Autodesk Inventor part; units mm, degrees
ref_plane "Work Plane1" through (-108.1719, 0, -146.2869) normal (0, 1, 0) x (0.6910823, 0, -0.7227761)
ref_plane "Work Plane2" through (-186.5657, -6, -277.4707) normal (0.6910823, 0, -0.7227761) x (0, 1, 0)
ref_plane "Work Plane3" through (-14.1966, -8.9, -56.4323) normal (-0.6910823, 0, 0.7227761) x (0.7227761, 0, 0.6910823)
sketch "Sketch1" plane through (0, 0, 0) normal (0, 1, 0) x (-1, 0, 0)
  line L0 (0, 0) -> (100, 0)
  line L1 (100, 0) -> (100, -50)
  line L2 (100, -50) -> (0, -50)
  line L3 (0, -50) -> (0, 0)
  dimension "d0" = 100
  dimension "d1" = 50
extrude "Extrusion1" add sketch "Sketch1" along normal blind 3
sketch "Sketch2" plane through (0, 3, 0) normal (0, 1, 0) x (1, 0, 0)
  circle A0 centre (-85, 25) radius 7
  circle A1 centre (-30, 25) radius 7
  line L0 (-100, 50) -> (-100, 0)
  line L1 (0, 0) -> (0, 50)
  line L2 (0, 50) -> (-100, 50)
  dimension "d4" = 14
  dimension "d5" = 14
  dimension "d6" = 15
  dimension "d7" = 30
  dimension "d8" = 25
  dimension "d9" = 25
extrude "Extrusion2" add sketch "Sketch2" along normal blind 18
sketch "Sketch3" plane through (-85, 21, -25) normal (0, 1, 0) x (1, 0, 0)
  circle A0 centre (0, 0) radius 7
  circle A1 centre (55, 0) radius 7
  circle A2 centre (0, 0) radius 2.875
  circle A3 centre (55, 0) radius 2.45
  point P0 (85, -25)
  dimension "d12" = 5.75
  dimension "d13" = 4.9
extrude "Extrusion3" add sketch "Sketch3" along normal blind 3 contours A2 | A3
sketch "Sketch5" plane through (-30, 24, -25) normal (0, 1, 0) x (1, 0, 0)
  circle A0 centre (0, 0) radius 1.925
  point P0 (30, -25)
  dimension "d20" = 3.85
extrude "Extrusion5" cut sketch "Sketch5" against normal up to surface (24 mm away)
sketch "Sketch7" plane through (0, 0, 0) normal (0, -1, 0) x (1, 0, 0)
  line L0 (2.4404, 5.5552) -> (-105.2601, 5.5552)
  line L1 (-105.2601, 5.5552) -> (-105.2601, -59.9514)
  line L2 (-105.2601, -59.9514) -> (2.4404, -59.9514)
  line L3 (2.4404, -59.9514) -> (2.4404, 5.5552)
  circle A0 centre (-30, -25) radius 2.45
  circle A1 centre (-30, -25) radius 7
  point P0 (0, 0)
extrude "Extrusion6" cut sketch "Sketch7" against normal blind 50 contours L3 L2 L1 L0
ref_plane "Work Plane1" through (-108.1719, 0, -146.2869) normal (0, 1, 0) x (0.6910823, 0, -0.7227761)
sketch "Sketch8" plane through (-108.1719, 0, -146.2869) normal (0, 1, 0) x (0.6910823, 0, -0.7227761)
  line L0 (-40.64, -147.32) -> (40.64, -147.32)
  line L1 (-40.64, 147.32) -> (-40.64, -147.32)
  line L2 (-43.34, -130.02) -> (-40.84, -130.02)
  line L3 (-40.84, -130.02) -> (-40.84, -150.02)
  line L4 (-40.84, -150.02) -> (-43.34, -150.02)
  line L5 (-43.34, -150.02) -> (-43.34, -130.02)
  line L6 (-23.34, -147.52) -> (-40.84, -147.52)
  line L7 (-40.84, -147.52) -> (-40.84, -150.02)
  line L8 (-23.34, -147.52) -> (-23.34, -150.02)
  line L9 (-23.34, -150.02) -> (-40.84, -150.02)
  line L10 (-40.84, -130.02) -> (-23.34, -130.02)
  line L11 (-23.34, -130.02) -> (-23.34, -147.52)
  arc A0 (-33.6873, -142.3194) -> (-35.0746, -141.7135) centre (-33.64, -140.32) ccw
  circle A1 centre (-33.64, -140.32) radius 3.8
  circle A2 centre (-33.64, -140.32) radius 7
  point P0 (-30.9769, -179.2803)
  point P1 (-40.84, -150.02)
  dimension "d26" = 0.2
  dimension "d27" = 0.2
  dimension "d29" = 20
  dimension "d30" = 2.5
  dimension "d31" = 2.5
  dimension "d32" = 20
extrude "Extrusion7" add sketch "Sketch8" along normal blind 2.5 contours L1 A2 L0 | L0 L11 L6 L3 L10 L1 | A2 L1 L10 L11 L0 | L8 L9 L3 L6 | L3 L4 L5 L2
sketch "Sketch9" plane through (0, 0, 0) normal (0, -1, 0) x (1, 0, 0)
  line L0 (-29.6926, -11.2856) -> (-15.8709, -25.7411)
  line L1 (-15.8709, -25.7411) -> (-17.6779, -27.4688)
  line L2 (-15.8709, -25.7411) -> (-30.3264, -39.5627)
  line L3 (-17.6779, -27.4688) -> (-31.4995, -13.0133)
  line L4 (-30.3264, -39.5627) -> (-44.1481, -25.1072)
  line L5 (-44.1481, -25.1072) -> (-42.4204, -26.9142)
  line L6 (-42.4204, -26.9142) -> (-29.7718, -14.8202)
  line L7 (-30.3264, -39.5627) -> (-44.1481, -25.1072)
  line L8 (-15.8709, -25.7411) -> (-30.3264, -39.5627)
  line L9 (-29.6926, -11.2856) -> (-15.8709, -25.7411)
  line L10 (-44.1481, -25.1072) -> (-29.6926, -11.2856)
  circle A0 centre (-30, -25) radius 1.925
  point P0 (0, 0)
  dimension "d35" = 2.5
  dimension "d36" = 0
  dimension "d37" = 2.5
extrude "Extrusion8" add sketch "Sketch9" along normal blind 6.4 contours L0 L1 L3 L10 | L3 L6 L4 L10
sketch "Sketch10" plane through (0, -6.4, 0) normal (0, -1, 0) x (1, 0, 0)
  line L0 (-30.3264, -39.5627) -> (-44.1481, -25.1072)
  line L1 (-44.1481, -25.1072) -> (-29.6926, -11.2856)
  line L2 (-29.6926, -11.2856) -> (-15.8709, -25.7411)
  line L3 (-15.8709, -25.7411) -> (-30.3264, -39.5627)
  circle A0 centre (-30, -25) radius 7
  circle A1 centre (-30, -25) radius 1.925
  point P0 (0, 0)
extrude "Extrusion9" add sketch "Sketch10" along normal blind 2.5 contours L0 L1 L2 L3 | A0
fillet "Fillet1" radius 2.5 1 edges at (-29.6926, -3.2, -11.2856)
fillet "Fillet2" radius 2.5 1 edges at (-37, 2.5, -25)
sketch "Sketch11" plane through (0, -8.9, 0) normal (0, -1, 0) x (1, 0, 0)
  circle A0 centre (-30, -25) radius 1.925
  arc A1 (-27.9649, -13.0925) -> (-31.4995, -13.0133) centre (-29.7718, -14.8202) ccw
  line L0 (-31.4995, -13.0133) -> (-44.1481, -25.1072)
  line L1 (-44.1481, -25.1072) -> (-30.3264, -39.5627)
  line L2 (-30.3264, -39.5627) -> (-15.8709, -25.7411)
  line L3 (-15.8709, -25.7411) -> (-27.9649, -13.0925)
  circle A2 centre (-30, -25) radius 2.45
  line L4 (-31.3275, -29.5443) -> (-34.5993, -26.1225)
  line L5 (-34.5993, -26.1225) -> (-33.2718, -21.5782)
  line L6 (-33.2718, -21.5782) -> (-28.6725, -20.4557)
  line L7 (-28.6725, -20.4557) -> (-25.4007, -23.8775)
  line L8 (-25.4007, -23.8775) -> (-26.7282, -28.4218)
  line L9 (-26.7282, -28.4218) -> (-31.3275, -29.5443)
  line L10 (-15.8709, -25.7411) -> (-27.9649, -13.0925)
  point P0 (0, 0)
  dimension "d44" = 8.2
extrude "Extrusion10" cut sketch "Sketch11" against normal blind 1.5 contours L4 L5 L6 L7 L8 L9
sketch "Sketch12" plane through (-30.3264, 0, -39.5627) normal (0.6910823, 0, -0.7227761) x (-0.7227761, 0, -0.6910823)
  line L0 (-17.5, 0) -> (0, 0)
  line L1 (0, 0) -> (0, 2.5)
  line L2 (-20, 2.5) -> (0, 2.5)
  line L3 (-20, -8.9) -> (-20, 2.5)
  line L4 (0, -8.9) -> (-20, -8.9)
  line L5 (0, -6.4) -> (0, -8.9)
  line L6 (0, -6.4) -> (-17.5, -6.4)
  line L7 (-17.5, 0) -> (-17.5, -6.4)
  point P0 (-49.2603, 0)
ref_plane "Work Plane2" through (-186.5657, -6, -277.4707) normal (0.6910823, 0, -0.7227761) x (0, 1, 0)
extrude "Extrusion11" add sketch "Sketch12" along normal blind 64.18
sketch "Sketch13" plane through (14.0272, 0, -85.9505) normal (0.6910823, 0, -0.7227761) x (-0.7227761, 0, -0.6910823)
  line L0 (0, 2.5) -> (-17.5, 2.5)
  line L1 (-17.5, -8.9) -> (0, -8.9)
  line L2 (0, -8.9) -> (0, 2.5)
  line L3 (-20, -8.9) -> (-20, 2.5)
  line L4 (-17.5, -6.4) -> (-17.5, 0)
  line L5 (-17.5, 0) -> (0, 0)
  line L6 (0, 0) -> (0, 2.5)
  line L7 (0, 2.5) -> (-20, 2.5)
  line L8 (-20, 2.5) -> (-20, -8.9)
  line L9 (-20, -8.9) -> (0, -8.9)
  line L10 (0, -8.9) -> (0, -6.4)
  line L11 (0, -6.4) -> (-17.5, -6.4)
  point P0 (-49.2603, 0)
  point P1 (-20, 2.5)
extrude "Extrusion12" add sketch "Sketch13" along normal blind 2.5
fillet "Fillet3" radius 2.5 1 edges at (30.2104, -3.2, -73.9358)
ref_plane "Work Plane3" through (-14.1966, -8.9, -56.4323) normal (-0.6910823, 0, 0.7227761) x (0.7227761, 0, 0.6910823)
mirror "Mirror1" about plane through (-14.1966, -8.9, -56.4323) normal (-0.6910823, 0, 0.7227761)
sketch "Sketch14" plane through (16.496, 24, -73.6284) normal (0, 1, 0) x (1, 0, 0)
  circle A0 centre (0, 0) radius 1.925
  circle A1 centre (0, 0) radius 1.925
  circle A2 centre (0, 0) radius 2.45
  point P0 (-16.496, -73.6284)
ref_plane "Work Plane4" through (-246.9785, 21, -281.7123) normal (0, -1, 0) x (0.7227761, 0, 0.6910823)
extrude "Extrusion13" cut sketch "Sketch14" against normal up to surface (3 mm away)
sketch "Sketch15" plane through (16.496, 21, -73.6284) normal (0, 1, 0) x (1, 0, 0)
  circle A0 centre (0, 0) radius 7
  point P0 (-16.496, -73.6284)
ref_plane "Work Plane5" through (-242.7369, 0, -277.4707) normal (0, 1, 0) x (-0.6910823, 0, 0.7227761)
extrude "Extrusion14" add sketch "Sketch15" against normal up to surface (21 mm away)
extrude "Extrusion15" cut sketch "Sketch11" against normal blind 1.5 contours A0 | A2 | L4 L5 L6 L7 L8 L9
extrude "Extrusion16" cut sketch "Sketch5" against normal up to surface (32.9 mm away)
properties part number "Base"
Build history of the part. All positions in model axes, mm. A direction names the side the tool comes from. Give positions to 0.01 mm unless a question says otherwise; leave off trailing zeros. Loops run counter-clockwise (first coordinate to the right, second up) from the corner with the lowest first, then second, coordinate; pieces in that order, holes last. Notation, with made-up numbers: (34, 5) -> (91, 5) arc R25 cw to (91, 28) -> close; hole circle Ø6 at (34, -25.75). An arc over 180 degrees is marked (long way). One line per question, with ' | ' between items. Start each with the question number.
1) Cut at A-A (x = -14.5). Give the cut face in (y, z).
2) Probe L1, parallel to Z at x = -30, y = 17.5 (3 decimals); L2, parallel to X at y = 15, z = -25 (3 decimals); L3, parallel to Y at x = -10.5, z = -46.5. List the from-to ranges inside material, lowest first.
3) Two-plate mould, pull along Y, no slides. Class faces 4 (the flat face through (-8, -6.4, -50)), 5 (the cylindrical face through (-27.663, 22.479, -24.264)), 6 (the flat face through (-7, -8.9, -49)): released by +Y, released by -Y, zero draft, split by the parting line, or undercut.
4) Cut at C-C (z = -36). Give the cut face in (x, y).
5) 3-axis set-ups, long thin cutter, end or side, ignore diameter. For faces 1 (the cylindrical face through (-26.77, 12.89, -31.21)), 2 (the flat face through (20.44, -3.16, -79.82)), 3 (the flat face through (-32.1, -7.4, -24.9)): which of +Z, -Z, +X, -X, +Y, -Y reach the whole face in a straight line?
6) Cut at B-B (y = 11.5). Give the cut face in (x, z) (3 decimals).
7) Pin check, flat tips, straight feed: pin 1 (8 mm diameter, centred on y = 8.5, z = -22, fed in from +X); pin 2 (4 mm diameter, centred on y = 9, z = -74.5, fed in from +X); pin 3 (1 mm diameter, centred on y = -4, z = -58.5, fed in from -X). Stop position of each tip, or through.
Return value:
1) outline: (-8.9, -56.11) -> (-6.4, -56.11) -> (-6.4, -30.79) -> (0, -30.79) -> (0, -56.12) -> (2.5, -56.11) -> (2.5, -27.17) -> (-8.9, -27.17) -> close
2) L1: -32 to -26.925, -23.075 to -18 | L2: -37 to -31.925, -28.075 to -23 | L3: -8.9 to -6.4, 0 to 2.5
3) face 4: undercut | face 5: zero draft | face 6: released by -Y
4) outline: (-33.73, -8.9) -> (-6.06, -8.9) -> (-6.06, 2.5) -> (-33.73, 2.5) -> (-33.73, 0) -> (-9.52, 0) -> (-9.52, -6.4) -> (-33.73, -6.4) -> close
5) face 1: +Y | face 2: -X | face 3: -Y
6) outline: circle Ø14 at (-30, -25); circle Ø14 at (16.496, -73.628); hole circle Ø3.85 at (-30, -25)
7) pin 1: x = -23 | pin 2: x = 23.5 | pin 3: x = 11.51
